Geometry check sheet. Reference: the model listing, model coordinates, mm. A direction names the side the tool comes from. Coordinates: 2 decimals unless noted, no trailing zeros. Write each loop counter-clockwise with the first axis right and the second up, starting at its lowest first coordinate (ties: lowest second). Pieces come first, ordered by that corner, then holes. Notation, with made-up numbers: (-4, 23) -> (18, 23) arc R11 ccw to (18, 44) -> close; hole circle Ø4 at (47.5, 63.25). An arc over 180 degrees is marked (long way). Answer in a Markdown table with one row per item. Add a question column.
1. Set-up check for faces 1 (the flat face through (-1, -13, 0)), 2 (the cylindrical face through (-1.92, -6.41, 0.03)), 3 (the cylindrical face through (-0.596, 0.493, 2.685)): record each of +Z, -Z, +X, -X, +Y, -Y from which the full face is reachable in a straight line by a thin tool's end or side.
2. Scan lines: L1, parallel to X at y = -11.25, z = -0.2; L2, parallel to Y at x = -1.7, z = -1.8; L3, parallel to Z at x = 1.3, y = -1. Record each from-to range of solid material in increasing order. Write a range as from..to.
3. Cross-section at B-B on y = -12.75. Record the cut outline in (x, z), and give its area (3 significant figures).
4. Cross-section at D-D on y = 5.5. Record the cut outline in (x, z).
5. Cross-section at C-C on x = 0. Record the cut outline in (y, z), and give its area (3 significant figures).
6. Mould release check, pull along X, two halves, no side actions. Record for faces 4 (the cylindrical face through (0.62, -9.37, 0.03)), 5 (the cylindrical face through (-0.5, 3.5, 2.4)), 6 (the flat face through (1, -19, 0)): pulls with the +X half, pulls with the -X half, needs draft (parallel to the pull), parting line crosses it, or undercut.
7. Cross-section at A-A on z = 0. Record the cut outline in (x, y).
8. Depth check by flat-ended pin: P1, Ø1.5, axis at y = -7.5, z = -0.5, coming from the -X side; P2, Ø1, axis at x = -1, z = 2, coming from the +Y side; P3, Ø1, axis at x = -1.5, z = 0, coming from the -Y side. Enter the tip coordinate at first touch or a pass-through.
```python
from build123d import *

# Parameters (mm, degrees)
CROQUIS1_R              = 2.75
SALIENTE_EXTRUIR1_DEPTH = 1
CROQUIS2_R              = 2.45
SALIENTE_EXTRUIR2_DEPTH = 5.05
C_PULA1_FACE_RADIUS     = 2.45
C_PULA1_HEIGHT          = 2.45
CROQUIS3_R              = 0.25
SALIENTE_EXTRUIR3_DEPTH = 16
CROQUIS5_R              = 0.25
SALIENTE_EXTRUIR5_DEPTH = 17
SKETCH2_R               = 0.25
CUT_EXTRUDE1_DEPTH      = 16
SKETCH3_R               = 0.25
CUT_EXTRUDE2_DEPTH      = 10
SKETCH4_R               = 0.65
BOSS_EXTRUDE1_DEPTH     = 13
SKETCH5_R               = 0.65
BOSS_EXTRUDE2_DEPTH     = 6


with BuildPart() as part:
    # Croquis1 → Saliente-Extruir1 (new body)
    with BuildSketch(Plane(origin=(0, 0, 0), x_dir=(1, 0, 0), z_dir=(0, 1, 0))):
        Circle(CROQUIS1_R)
    extrude(amount=SALIENTE_EXTRUIR1_DEPTH)

    # Croquis2 → Saliente-Extruir2 (add)
    with BuildSketch(Plane(origin=(0, 1, 0), x_dir=(1, 0, 0), z_dir=(0, 1, 0))):
        Circle(CROQUIS2_R)
    extrude(amount=SALIENTE_EXTRUIR2_DEPTH)

    # Cúpula1: a dome of height H over a round flat face of radius A is a cap of a sphere of radius (A * A + H * H) / (2 * H)
    c_pula1_r = (C_PULA1_FACE_RADIUS * C_PULA1_FACE_RADIUS + C_PULA1_HEIGHT * C_PULA1_HEIGHT) / (2 * C_PULA1_HEIGHT)
    c_pula1_base = Plane((0, 6.05, 0), z_dir=(0, 1, 0))
    with Locations(c_pula1_base.offset(C_PULA1_HEIGHT - c_pula1_r)):
        c_pula1_ball = Sphere(c_pula1_r, mode=Mode.PRIVATE)
    add(split(c_pula1_ball, bisect_by=c_pula1_base, keep=Keep.TOP, mode=Mode.PRIVATE))

    # Croquis3 → Saliente-Extruir3 (add)
    with BuildSketch(Plane.XZ):
        with Locations((-1.205162028, 0)):
            Circle(CROQUIS3_R)
    extrude(amount=SALIENTE_EXTRUIR3_DEPTH)

    # Croquis5 → Saliente-Extruir5 (add)
    with BuildSketch(Plane.XZ):
        with Locations((1.205162028, 0)):
            Circle(CROQUIS5_R)
    extrude(amount=SALIENTE_EXTRUIR5_DEPTH)

    # Sketch2 → Cut-Extrude1 (cut)
    with BuildSketch(Plane.XZ.offset(16)):
        with Locations((-1.205162028, 0)):
            Circle(SKETCH2_R)
        with Locations((1.205162028, 0)):
            Circle(SKETCH2_R)
    extrude(amount=-CUT_EXTRUDE1_DEPTH, mode=Mode.SUBTRACT)

    # Sketch3 → Cut-Extrude2 (cut)
    with BuildSketch(Plane.XZ.offset(17)):
        with Locations((1.205162028, 0)):
            Circle(SKETCH3_R)
    extrude(amount=-CUT_EXTRUDE2_DEPTH, mode=Mode.SUBTRACT)

    # Sketch4 → Boss-Extrude1 (add)
    with BuildSketch(Plane.XZ):
        with Locations((1.27, 0)):
            Circle(SKETCH4_R)
        with Locations((-1.27, 0)):
            Circle(SKETCH4_R)
    extrude(amount=BOSS_EXTRUDE1_DEPTH)

    # Sketch5 → Boss-Extrude2 (add)
    with BuildSketch(Plane.XZ.offset(13)):
        with Locations((1.27, 0)):
            Circle(SKETCH5_R)
    extrude(amount=BOSS_EXTRUDE2_DEPTH)


solid = part.part
```
Results found:
| question | item | result |
|---|---|---|
| 1 | face 1 | +Z, -Z, -X, -Y |
| 1 | face 2 | -Y |
| 1 | face 3 | +Y, -Y |
| 2 | L1 | x = -1.89..-0.65, 0.65..1.89 |
| 2 | L2 | y = 0..1 |
| 2 | L3 | z = -0.65..0.65 |
| 3 | outline | circle Ø1.3 at (-1.27, 0); circle Ø1.3 at (1.27, 0) |
| 3 | area | 2.65 mm^2 |
| 4 | outline | circle Ø4.9 at (0, 0) |
| 5 | outline | (0, -2.75) -> (1, -2.75) -> (1, -2.45) -> (6.05, -2.45) arc R2.45 ccw to (6.05, 2.45) -> (1, 2.45) -> (1, 2.75) -> (0, 2.75) -> close |
| 5 | area | 39.7 mm^2 |
| 6 | face 4 | undercut |
| 6 | face 5 | parting line crosses it |
| 6 | face 6 | needs draft |
| 7 | outline | (-2.75, 0) -> (-1.92, 0) -> (-1.92, -13) -> (-0.62, -13) -> (-0.62, 0) -> (0.62, 0) -> (0.62, -19) -> (1.92, -19) -> (1.92, 0) -> (2.75, 0) -> (2.75, 1) -> (2.45, 1) -> (2.45, 6.05) arc R2.45 ccw to (-2.45, 6.05) -> (-2.45, 1) -> (-2.75, 1) -> close |
| 8 | P1 | stops at x = -1.92 |
| 8 | P2 | stops at y = 7.78 |
| 8 | P3 | stops at y = -13 |
